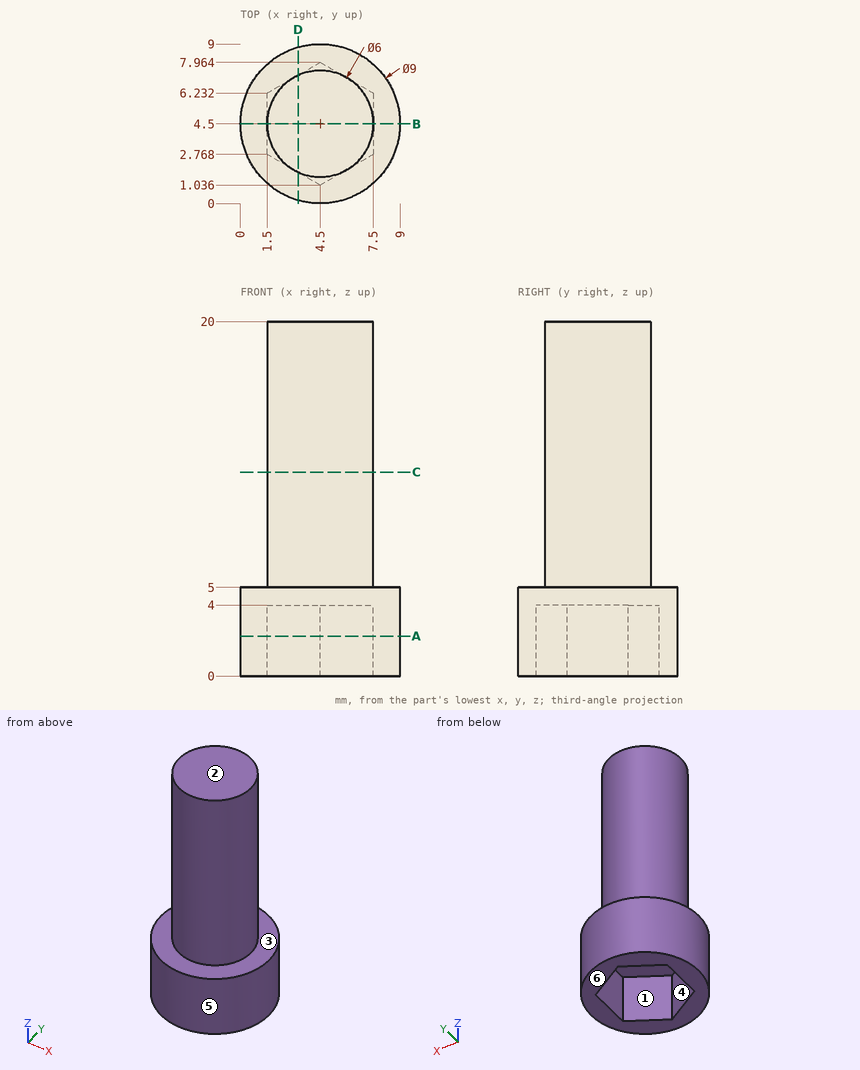
For this review, use the dimensioned drawing (mm, ordinates from the lowest corner) and the shaded views. A direction names the side the tool comes from. Round coordinates to 2 decimals unless told otherwise and drop trailing zeros. Order: outer loops, then holes, each group sorted by start corner. A loop starts at its lowest first (then second) coordinate and runs counter-clockwise, first axis right, second up.
1) Consider section A-A (z = 2.25). State the section outline as (x, y) points.
The answers:
outline: circle Ø9 at (4.5, 4.5); hole (1.5, 2.77) - (4.5, 1.04) - (7.5, 2.77) - (7.5, 6.23) - (4.5, 7.96) - (1.5, 6.23) - close
2) Clearance check with a flat-ended pin moving along its axis: pin 1 Ø2 at (y, z) = (4, 13) entering from -X. State where the tip first meets the part, or that it passes through.
The answers:
pin 1: stops at x = 1.5
3) For L1, parallel to Z at x = 6.25, y = 6.5; L2, parallel to Z at x = 1.5, y = 7.75; L3, parallel to Y at x = 3, z = 2, list the stretches that pass through material, from the lowest coordinate up.
The answers:
L1: z = 4 to 20
L2: z = 0 to 5
L3: y = 0.26 to 1.9, 7.1 to 8.74
4) Consider section B-B (y = 4.5). State the section outline as (x, z) points.
The answers:
outline: (0, 0) - (1.5, 0) - (1.5, 4) - (7.5, 4) - (7.5, 0) - (9, 0) - (9, 5) - (7.5, 5) - (7.5, 20) - (1.5, 20) - (1.5, 5) - (0, 5) - close
5) Draft analysis for pull direction X (two halves, no side actions). For the marked faces 4, 5 and 6, state which applies: released by +X, released by -X, zero draft, split by the parting line, or undercut.
The answers:
face 4: undercut
face 5: split by the parting line
face 6: zero draft
6) Machinability: for the marked faces 1, 2 and 3, which of the approach directions +Z, -Z, +X, -X, +Y, -Y give a long, thin tool a straight path to every point of the face, cutting with its end or side? Answer none if there is none.
The answers:
face 1: -Z
face 2: +Z, +X, -X, +Y, -Y
face 3: +Z
7) Consider section D-D (x = 3.25). State the section outline as (y, z) points.
The answers:
outline: (0.18, 0) - (1.76, 0) - (1.76, 4) - (7.24, 4) - (7.24, 0) - (8.82, 0) - (8.82, 5) - (7.23, 5) - (7.23, 20) - (1.77, 20) - (1.77, 5) - (0.18, 5) - close
8) Consider section C-C (z = 11.5). State the section outline as (x, y) points.
The answers:
outline: circle Ø6 at (4.5, 4.5)
